The listing builds one solid part. Answer for the finished solid, in the listing's coordinates (mm). A direction names the side the tool comes from. Coordinates: 2 decimals unless noted, no trailing zeros. Loops run counter-clockwise (first coordinate to the right, second up) from the corner with the lowest first, then second, coordinate; pieces in that order, holes last. Notation, with made-up numbers: (83.5, 15) -> (98.5, 15) arc R23 cw to (98.5, 24) -> close; hole circle Ø11 at (35, 64.5). An arc over 180 degrees is marked (long way). Answer in a Markdown table with one row per item.
```python
from build123d import *

# Parameters (mm, degrees)
F0_R     = 10
F0_R_2   = 8
F1_DEPTH = 6
F2_R     = 10
F2_W     = 0.8
F2_H     = 2
F2_W_2   = 5
F3_DEPTH = 1
F4_DEPTH = 1.5


with BuildPart() as f1:
    # F0 (on Top) → F1 (new body)
    with BuildSketch(Plane.XY):
        Circle(F0_R)
        Circle(F0_R_2, mode=Mode.SUBTRACT)
    extrude(amount=F1_DEPTH)

    # F2 (on Top) → F3 (join)
    with BuildSketch(Plane.XY):
        Circle(F2_R)
        with Locations((-9, 0)):
            Rectangle(F2_W, F2_H, mode=Mode.SUBTRACT)
        Rectangle(F2_W_2, F2_H, mode=Mode.SUBTRACT)
        with Locations((9, 0)):
            Rectangle(F2_W, F2_H, mode=Mode.SUBTRACT)
    extrude(amount=F3_DEPTH)

    # F2 (on Top) → F4 (cut)
    with BuildSketch(Plane.XY):
        with Locations((9, 0)):
            Rectangle(F2_W, F2_H)
        with Locations((-9, 0)):
            Rectangle(F2_W, F2_H)
    extrude(amount=F4_DEPTH, mode=Mode.SUBTRACT)


solid = f1.part
```
Item 1: Flat-ended cylindrical pins translate along their axes: pin 1 Ø1 at (y, z) = (6.5, 2) entering from -X; pin 2 Ø0.6 at (x, z) = (9, 0.5) entering from +Y; pin 3 Ø2 at (x, z) = (3, 1.5) entering from -Y. Find the tip coordinate at first contact, or state that the pin passes through.
Findings below:
| item | result |
|---|---|
| pin 1 | stops at x = -8 |
| pin 2 | stops at y = 4.93 |
| pin 3 | stops at y = -9.8 |
Item 2: A cutting plane is placed at D-D, the plane y = 6. Determine the outline of the cut face in (x, z), plus the area to 3 significant figures.
Findings below:
| item | result |
|---|---|
| outline | (-8, 0) -> (8, 0) -> (8, 6) -> (5.29, 6) -> (5.29, 1) -> (-5.29, 1) -> (-5.29, 6) -> (-8, 6) -> close |
| area | 43.1 mm2 |
Item 3: A cutting plane is placed at B-B, the plane x = 0. Determine the outline of the cut face in (y, z), plus the area to 3 significant figures.
Findings below:
| item | result |
|---|---|
| outline | (-10, 0) -> (-1, 0) -> (-1, 1) -> (-8, 1) -> (-8, 6) -> (-10, 6) -> close; (1, 0) -> (10, 0) -> (10, 6) -> (8, 6) -> (8, 1) -> (1, 1) -> close |
| area | 38.0 mm2 |
Item 4: A cutting plane is placed at C-C, the plane z = 5.15. Determine the outline of the cut face in (x, y), plus the area to 3 significant figures.
Findings below:
| item | result |
|---|---|
| outline | circle Ø20 at (0, 0); hole circle Ø16 at (0, 0) |
| area | 113 mm2 |
Item 5: Determine the mould class of faces 4 (the face through (-2.17, -9.76, 2.96)), 5 (the face through (0, 8.2, 6)), 6 (the face through (-9, -1, 1)) for opening direction X: +X half, -X half, draft (parallel to the pull), parting line (faces both ways), or undercut.
Findings below:
| item | result |
|---|---|
| face 4 | parting line |
| face 5 | draft |
| face 6 | undercut |
Item 6: Find the intervals of material crossed by probe 1 along Y at (x, z) = (0, 3.6); probe 2 along Z at (x, y) = (1.25, -1.25); probe 3 along Z at (x, y) = (9.25, -0.75), in increasing order.
Findings below:
| item | result |
|---|---|
| probe 1 | y = -10 to -8, 8 to 10 |
| probe 2 | z = 0 to 1 |
| probe 3 | z = 1.5 to 6 |
Item 7: A cutting plane is placed at A-A, the plane y = 0. Determine the outline of the cut face in (x, z).
Findings below:
| item | result |
|---|---|
| outline | (-10, 0) -> (-9.4, 0) -> (-9.4, 1.5) -> (-8.6, 1.5) -> (-8.6, 0) -> (-2.5, 0) -> (-2.5, 1) -> (-8, 1) -> (-8, 6) -> (-10, 6) -> close; (2.5, 0) -> (8.6, 0) -> (8.6, 1.5) -> (9.4, 1.5) -> (9.4, 0) -> (10, 0) -> (10, 6) -> (8, 6) -> (8, 1) -> (2.5, 1) -> close |
Item 8: A tool of negligible diameter and unlimited length cuts with its end or side. For faces 1 (the face through (0, -2, 1)), 2 (the face through (2.5, 0, 0.5)), 3 (the face through (-8.6, 0, 1)), from which of +Z, -Z, +X, -X, +Y, -Y can it reach the whole face along a straight path? Write none if from no direction.
Findings below:
| item | result |
|---|---|
| face 1 | +Z |
| face 2 | +Z, -Z |
| face 3 | -Z |
